```python
from build123d import *

# Parameters (mm, degrees)
SKETCH1_R           = 100
BOSS_EXTRUDE1_DEPTH = 150
SKETCH4_R           = 62.5
SKETCH4_R_2         = 50
BOSS_EXTRUDE3_DEPTH = 500


with BuildPart() as part:
    # Sketch1 → Boss-Extrude1 (new body)
    with BuildSketch(Plane(origin=(0, 0, 0), x_dir=(1, 0, 0), z_dir=(0, 1, 0))):
        with BuildLine():
            Line((-125, 175), (125, 175))
            ThreePointArc((125, 175), (160.355339059, 160.355339059), (175, 125))
            Line((175, 125), (175, -125))
            ThreePointArc((175, -125), (160.355339059, -160.355339059), (125, -175))
            Line((125, -175), (-125, -175))
            ThreePointArc((-125, -175), (-160.355339059, -160.355339059), (-175, -125))
            Line((-175, -125), (-175, 125))
            ThreePointArc((-175, 125), (-160.355339059, 160.355339059), (-125, 175))
        make_face()
        with Locations(Location((0, 0, 0), (0, 0, 270))):
            Circle(SKETCH1_R, mode=Mode.SUBTRACT)
    extrude(amount=BOSS_EXTRUDE1_DEPTH)

    # Sketch4 → Boss-Extrude3 (add)
    with BuildSketch(Plane.XY.offset(175)):
        with Locations(Location((0, 75, 0), (0, 0, 180))):
            Circle(SKETCH4_R)
        with Locations((0, 75)):
            Circle(SKETCH4_R_2, mode=Mode.SUBTRACT)
    extrude(amount=BOSS_EXTRUDE3_DEPTH)


solid = part.part
```
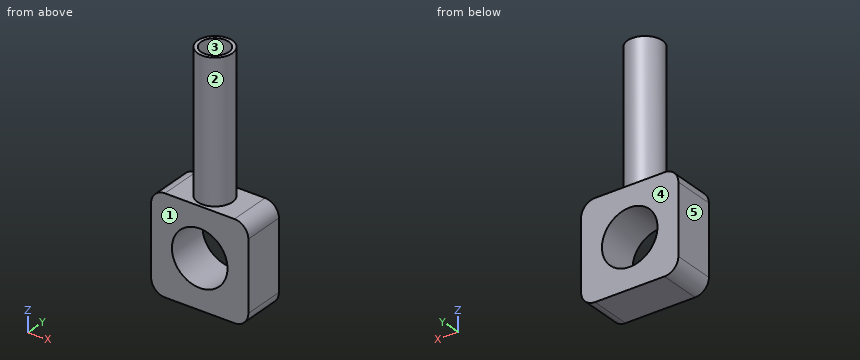
Geometry: final body of the model. Coordinates: model frame, mm. Face numbers are marked on the shaded views. A direction names the side the tool comes from. Coordinates: 2 decimals unless noted, no trailing zeros. Order: outer loops, then holes, each group sorted by start corner. A loop starts at its lowest first (then second) coordinate and runs counter-clockwise, first axis right, second up. Notation, with made-up numbers: M -33.5,66.25 L -0.5,66.25 A22 ccw -0.5,82.25 Z; hole C -15,-18 d8. An arc over 180 degrees is marked long. Answer as CSV lines item,"result".
Q1. Section B-B on x = 0. Return the cut outline in (y, z).
Answers:
outline,"M 0,-175 L 150,-175 L 150,-100 L 0,-100 Z; M 0,100 L 150,100 L 150,175 L 137.5,175 L 137.5,675 L 125,675 L 125,175 L 25,175 L 25,675 L 12.5,675 L 12.5,175 L 0,175 Z"
Q2. Set-up query: the marked faces 1 and 2. Return all of +Z, -Z, +X, -X, +Y, -Y with unobstructed straight access to the full face (end or side cutting, diameter ignored); none if empty.
Answers:
face 1,"+Z, -Z, +X, -X, -Y"
face 2,"+Z"
Q3. Section D-D on x = -79.5. Return the cut outline in (y, z).
Answers:
outline,"M 0,-175 L 150,-175 L 150,-60.66 L 0,-60.66 Z; M 0,60.66 L 150,60.66 L 150,175 L 0,175 Z"
Q4. Section C-C on y = 75. Return the cut outline in (x, z), and give its area (3 significant figures).
Answers:
outline,"M -175,-125 A50 ccw -125,-175 L 125,-175 A50 ccw 175,-125 L 175,125 A50 ccw 125,175 L 62.5,175 L 62.5,675 L 50,675 L 50,175 L -50,175 L -50,675 L -62.5,675 L -62.5,175 L -125,175 A50 ccw -175,125 Z; hole C 0,0 d200"
area,"101,000 mm^2"
Q5. First-contact query: P1, Ø1, axis at y = 92, z = 253, coming from the +X side; P2, Ø6, axis at x = -56, z = 216, coming from the -Y side; P3, Ø4, axis at y = 47.5, z = 523.5, coming from the -X side. Flat tips, straight axial feed; report the tip coordinate or a pass-through.
Answers:
P1,"stops at x = 60.28"
P2,"stops at y = 41.88"
P3,"stops at x = -57.06"
Q6. Section A-A on z = 0. Return the cut outline in (x, y), and give its area (3 significant figures).
Answers:
outline,"M -175,0 L -100,0 L -100,150 L -175,150 Z; M 100,0 L 175,0 L 175,150 L 100,150 Z"
area,"22,500 mm^2"
Q7. Draft query along X for the marked faces 3, 4 and 5. Return one class per face: pulls with the +X half, pulls with the -X half, needs draft (parallel to the pull), parting line crosses it, or undercut.
Answers:
face 3,"undercut"
face 4,"needs draft"
face 5,"pulls with the -X half"
Q8. Line query: probe 1 along X at (y, z) = (96, 0); probe 2 along Y at (x, z) = (0, 459.5); probe 3 along X at (y, z) = (43, 370). Output: solid intervals per line, ascending. Write a range as [from, to].
Answers:
probe 1,"x = [-175, -100], [100, 175]"
probe 2,"y = [12.5, 25], [125, 137.5]"
probe 3,"x = [-53.69, -38.42], [38.42, 53.69]"
